CAD build for the part. Positions are in the model's coordinates, mm. Face numbers are marked on the shaded views. A direction names the side the tool comes from. Round coordinates to 2 decimals unless told otherwise and drop trailing zeros. Order: outer loops, then holes, each group sorted by start corner. A loop starts at its lowest first (then second) coordinate and runs counter-clockwise, first axis right, second up. Notation, with made-up numbers: M 77.5,17.25 L 121.5,17.25 A7 cw 121.5,26.25 Z; hole C 33.5,50 d9. An arc over 180 degrees is marked long. Answer as a JSON object with one key per item and string values.
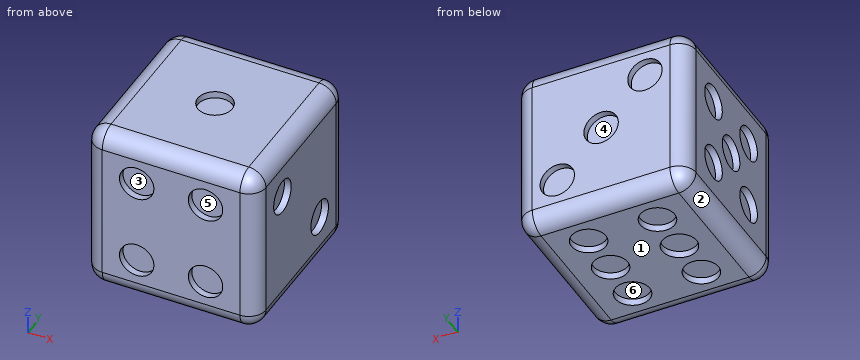
```python
from build123d import *

# Parameters (mm, degrees)
F0_W      = 50
F0_H      = 50
F1_DEPTH  = 50
F2_R      = 5
F3_DEPTH  = 2
F4_R      = 5
F5_DEPTH  = 2
F6_R      = 5
F7_DEPTH  = 2
F8_R      = 5
F9_DEPTH  = 2
F10_R     = 5
F11_DEPTH = 2
F12_R     = 5
F13_DEPTH = 2
F14_R     = 5


with BuildPart() as f1:
    # F0 (on Top) → F1 (new body)
    with BuildSketch(Plane.XY):
        Rectangle(F0_W, F0_H)
    extrude(amount=F1_DEPTH)

    # F2 (on face) → F3 (cut)
    with BuildSketch(Plane.XY.offset(50)):
        Circle(F2_R)
    extrude(amount=-F3_DEPTH, mode=Mode.SUBTRACT)

    # F4 (on face) → F5 (cut)
    with BuildSketch(Plane.YZ.offset(25)):
        with Locations((10.606602, 14.393398)):
            Circle(F4_R)
        with Locations((-10.606602, 35.606602)):
            Circle(F4_R)
    extrude(amount=-F5_DEPTH, mode=Mode.SUBTRACT)

    # F6 (on face) → F7 (cut)
    with BuildSketch(Plane(origin=(0, 0, 0), x_dir=(1, 0, 0), z_dir=(0, 0, -1))):
        with Locations((10, -12.5)):
            Circle(F6_R)
        with Locations((10, 0)):
            Circle(F6_R)
        with Locations((10, 12.5)):
            Circle(F6_R)
        with Locations((-10, -12.5)):
            Circle(F6_R)
        with Locations((-10, 0)):
            Circle(F6_R)
        with Locations((-10, 12.5)):
            Circle(F6_R)
    extrude(amount=-F7_DEPTH, mode=Mode.SUBTRACT)

    # F8 (on face) → F9 (cut)
    with BuildSketch(Plane(origin=(0, 25, 0), x_dir=(-1, 0, 0), z_dir=(0, 1, 0))):
        with Locations((-12.727922, 12.272078)):
            Circle(F8_R)
        with Locations((0, 25)):
            Circle(F8_R)
        with Locations((12.727922, 37.727922)):
            Circle(F8_R)
    extrude(amount=-F9_DEPTH, mode=Mode.SUBTRACT)

    # F10 (on face) → F11 (cut)
    with BuildSketch(Plane.XZ.offset(25)):
        with Locations((-10, 37.5)):
            Circle(F10_R)
        with Locations((-10, 12.5)):
            Circle(F10_R)
        with Locations((10, 12.5)):
            Circle(F10_R)
        with Locations((10, 37.5)):
            Circle(F10_R)
    extrude(amount=-F11_DEPTH, mode=Mode.SUBTRACT)

    # F12 (on face) → F13 (cut)
    with BuildSketch(Plane(origin=(-25, 0, 0), x_dir=(0, -1, 0), z_dir=(-1, 0, 0))):
        with Locations((-10, 35)):
            Circle(F12_R)
        with Locations((0, 25)):
            Circle(F12_R)
        with Locations((10, 35)):
            Circle(F12_R)
        with Locations((10, 15)):
            Circle(F12_R)
        with Locations((-10, 15)):
            Circle(F12_R)
    extrude(amount=-F13_DEPTH, mode=Mode.SUBTRACT)

    # F14
    f14_edges = [f1.edges().sort_by_distance(p)[0] for p in [
        (25, 0, 50),
        (25, -25, 25),
        (-25, -25, 25),
        (0, 25, 0),
        (-25, 25, 25),
        (-25, 0, 50),
        (25, 0, 0),
        (0, -25, 0),
        (25, 25, 25),
        (-25, 0, 0),
        (0, 25, 50),
        (0, -25, 50),
    ]]
    fillet(f14_edges, radius=F14_R)


solid = f1.part
```
Item 1: Saw through at C-C on z = 25. List the corners of the cut face in (x, y).
Worked answers:
{"outline": "M -25,-20 A5 ccw -20,-25 L 20,-25 A5 ccw 25,-20 L 25,20 A5 ccw 20,25 L 5,25 L 5,23 L -5,23 L -5,25 L -20,25 A5 ccw -25,20 L -25,5 L -23,5 L -23,-5 L -25,-5 Z"}
Item 2: 3-axis set-ups, long thin cutter, end or side, ignore diameter. For the marked faces 4, 5 and 6: which of +Z, -Z, +X, -X, +Y, -Y reach the whole face in a straight line?
Worked answers:
{"face 4": "+Y", "face 5": "-Y", "face 6": "-Z"}
Item 3: Drop flat-ended pins along their axis: pin 1 Ø8 at (x, z) = (10, 12.5) entering from +Y; pin 2 Ø8 at (y, z) = (10, 15) entering from +X; pin 3 Ø8 at (x, y) = (10, -12.5) entering from -Z; pin 4 Ø9 at (y, z) = (-10, 15) entering from -X. Give the stop position or say it passes through.
Worked answers:
{"pin 1": "stops at y = 25", "pin 2": "stops at x = 23", "pin 3": "stops at z = 2", "pin 4": "stops at x = -23"}
Item 4: Two-plate mould, pull along X, no slides. Class the marked faces 1, 2 and 3: released by +X, released by -X, zero draft, split by the parting line, or undercut.
Worked answers:
{"face 1": "zero draft", "face 2": "released by -X", "face 3": "undercut"}
Item 5: Saw through at A-A on x = 0. List the corners of the cut face in (y, z).
Worked answers:
{"outline": "M -25,5 A5 ccw -20,0 L 20,0 A5 ccw 25,5 L 25,20 L 23,20 L 23,30 L 25,30 L 25,45 A5 ccw 20,50 L 5,50 L 5,48 L -5,48 L -5,50 L -20,50 A5 ccw -25,45 Z"}
Item 6: Saw through at B-B on y = 0. List the corners of the cut face in (x, z).
Worked answers:
{"outline": "M -25,5 A5 ccw -20,0 L -15,0 L -15,2 L -5,2 L -5,0 L 5,0 L 5,2 L 15,2 L 15,0 L 20,0 A5 ccw 25,5 L 25,45 A5 ccw 20,50 L 5,50 L 5,48 L -5,48 L -5,50 L -20,50 A5 ccw -25,45 L -25,30 L -23,30 L -23,20 L -25,20 Z"}
Item 7: Wall check: line 1 along Y through (x, z) = (10, 1); line 2 along Z through (x, y) = (-24, 10); line 3 along Z through (x, y) = (10, -10). Give the ranges that are in metal, low to high. Write a range as [from, to].
Worked answers:
{"line 1": "y = [-23, -17.5], [-7.5, -5], [5, 7.5], [17.5, 23]", "line 2": "z = [2, 10], [20, 30], [40, 48]", "line 3": "z = [2, 50]"}
